from build123d import *

# Parameters (mm, degrees)
F0_R            = 140.462
F1_DEPTH        = 25.4
F3_DEPTH        = 50.801
F3_COPIES_COUNT = 10
F6_DEPTH        = 50.801
F6_COPIES_COUNT = 5
F7_R            = 12.7
F8_DEPTH        = 50.801


# Not quite as in the source:
# - a pattern or mirror of a feature is missing from the dataset's text; its kind, count and spacing are read off the source's solid


with BuildPart() as f1:
    # F0 (on Top) → F1 (new body, symmetric)
    with BuildSketch(Plane.XY):
        Circle(F0_R)
    extrude(amount=F1_DEPTH, both=True)

    # F2 (on face) → F3 (cut, through all)
    with BuildSketch(Plane.XY.offset(25.4)):
        with BuildLine():
            ThreePointArc((-19.05, 94.9452416198), (0, 96.8375), (19.05, 94.9452416198))
            Line((19.05, 94.9452416198), (19.05, 139.1641870023))
            ThreePointArc((19.05, 139.1641870023), (0, 140.462), (-19.05, 139.1641870023))
            Line((-19.05, 139.1641870023), (-19.05, 94.9452416198))
        make_face()
    f3 = extrude(amount=-F3_DEPTH, mode=Mode.SUBTRACT)

    # F3_copies: F3 ×10 about axis
    f3_copies_axis = Axis((0, 0, 0), (0, 0, 1))
    for i in range(1, F3_COPIES_COUNT):
        add(f3.rotate(f3_copies_axis, i * 360 / F3_COPIES_COUNT), mode=Mode.SUBTRACT)

    # F5 (on face) → F6 (cut, through all)
    with BuildSketch(Plane.XY.offset(25.4)):
        with BuildLine():
            ThreePointArc((71.7178399755, 30.4867595727), (75.6356515828, 34.1286194106), (75.3810322275, 39.4716110682))
            ThreePointArc((75.3810322275, 39.4716110682), (50.0146471176, 68.8392560514), (14.2457129032, 83.8890205204))
            ThreePointArc((14.2457129032, 83.8890205204), (9.0855441629, 82.4801026945), (6.8326, 77.6286458547))
            Line((6.8326, 77.6286458547), (6.8326, 18.1442923048))
            ThreePointArc((6.8326, 18.1442923048), (9.4501636479, 13.0070343905), (15.1448579143, 12.1050834263))
            Line((15.1448579143, 12.1050834263), (71.7178399755, 30.4867595727))
        make_face()
    f6 = extrude(amount=-F6_DEPTH, mode=Mode.SUBTRACT)

    # F6_copies: F6 ×5 about axis
    f6_copies_axis = Axis((0, 0, 0), (0, 0, 1))
    for i in range(1, F6_COPIES_COUNT):
        add(f6.rotate(f6_copies_axis, i * 360 / F6_COPIES_COUNT), mode=Mode.SUBTRACT)

    # F7 (on face) → F8 (cut, through all)
    with BuildSketch(Plane.XY.offset(25.4)):
        Circle(F7_R)
    extrude(amount=-F8_DEPTH, mode=Mode.SUBTRACT)


solid = f1.part
Can you work these out from the model? Positions are in its coordinate system, mm. A direction names the side the tool comes from. Round coordinates to 2 decimals unless told otherwise and drop trailing zeros. Write each loop counter-clockwise with the first axis right and the second up, starting at its lowest first coordinate (ties: lowest second). Pieces come first, ordered by that corner, then holes. Notation, with made-up numbers: (-5.5, 31) -> (34.5, 31) arc R20 ccw to (34.5, 48) -> close; hole circle Ø10 at (-0.75, 84). An arc over 180 degrees is marked (long way). One line per question, with ' | ' between items. Start each with the question number.
1) If we mould it in two halves opening along Y, with no side actions, what happens to faces 4 (the flat face through (116.92, 17.96, 0.36)), 5 (the cylindrical face through (-140.46, 0.35, 0.36)), 6 (the flat face through (19.05, 117, 0))? For each: released by +Y, released by -Y, zero draft, split by the parting line, or undercut.
2) Suppose I cut it at D-D on x = 46.5. Write out the boundary of the cut face in (y, z).
3) I'm going to push flat-ended pins straight in: P1, Ø10, axis at x = -62, z = -14.5, coming from the +Y side; P2, Ø3, axis at x = -109, y = -19, coming from the -Z side; P3, Ø5, axis at y = -20, z = -18, coming from the +X side; P4, Ø1, axis at y = 6, z = 20, coming from the +X side. Where does each tip first touch, or does it pass through?
4) I need wall thicknesses on line 1 (Y direction, x = 0, z = 8); line 2 (Y direction, x = 65, z = -15); line 3 (X direction, y = -37.5, z = -12.5). Which ranges of each line are inside material? Lowest first, please. Write a range as [from, to].
5) Suppose I cut it at C-C on y = 107.5. Write out the boundary of the cut face in (x, z).
6) Suppose I cut it at B-B on y = -55.5. Write out the boundary of the cut face in (x, z), then the cut area to 3 significant figures.
7) On a 3-axis mill with a long thin cutter (end or side, diameter ignored), from which of +Z, -Z, +X, -X, +Y, -Y can I reach the whole of each face in a straight line? I mean faces 1 (the flat face through (-19.05, 117, 0)), 2 (the flat face through (105.733, 54.385, 0.356)), 3 (the cylindrical face through (-41.15, -71.99, 0.36)). Say none if no direction works.
8) Suppose I cut it at A-A on x = 0. Write out the boundary of the cut face in (y, z), then the cut area to 3 significant figures.
Return value:
1) face 4: undercut | face 5: split by the parting line | face 6: zero draft
2) outline: (-132.54, -25.4) -> (-96.41, -25.4) -> (-96.41, 25.4) -> (-132.54, 25.4) -> close; (-84.94, -25.4) -> (-52.38, -25.4) -> (-52.38, 25.4) -> (-84.94, 25.4) -> close; (7.92, -25.4) -> (22.29, -25.4) -> (22.29, 25.4) -> (7.92, 25.4) -> close; (71.26, -25.4) -> (84.94, -25.4) -> (84.94, 25.4) -> (71.26, 25.4) -> close; (96.41, -25.4) -> (132.54, -25.4) -> (132.54, 25.4) -> (96.41, 25.4) -> close
3) P1: stops at y = 128.38 | P2: passes through | P3: stops at x = 139.37 | P4: stops at x = 140.35
4) line 1: y = [-96.84, -85.09], [-16.08, -12.7], [12.7, 96.84] | line 2: y = [-124.52, -121.87], [-71.78, -54.91], [13.94, 28.3], [54.91, 71.78], [121.87, 124.52] | line 3: x = [-89.28, -76.38], [-35.69, -18.8], [18.8, 35.69], [76.38, 89.28]
5) outline: (-54.56, -25.4) -> (-19.05, -25.4) -> (-19.05, 25.4) -> (-54.56, 25.4) -> close; (19.05, -25.4) -> (54.56, -25.4) -> (54.56, 25.4) -> (19.05, 25.4) -> close
6) outline: (-109.16, -25.4) -> (-64.5, -25.4) -> (-64.5, 25.4) -> (-109.16, 25.4) -> close; (-48.77, -25.4) -> (-31.88, -25.4) -> (-31.88, 25.4) -> (-48.77, 25.4) -> close; (31.88, -25.4) -> (48.77, -25.4) -> (48.77, 25.4) -> (31.88, 25.4) -> close; (64.5, -25.4) -> (109.16, -25.4) -> (109.16, 25.4) -> (64.5, 25.4) -> close | area: 6,250 mm2
7) face 1: +Z, -Z, +Y | face 2: +Z, -Z, +X | face 3: +Z, -Z
8) outline: (-96.84, -25.4) -> (-85.09, -25.4) -> (-85.09, 25.4) -> (-96.84, 25.4) -> close; (-16.08, -25.4) -> (-12.7, -25.4) -> (-12.7, 25.4) -> (-16.08, 25.4) -> close; (12.7, -25.4) -> (96.84, -25.4) -> (96.84, 25.4) -> (12.7, 25.4) -> close | area: 5,040 mm2
